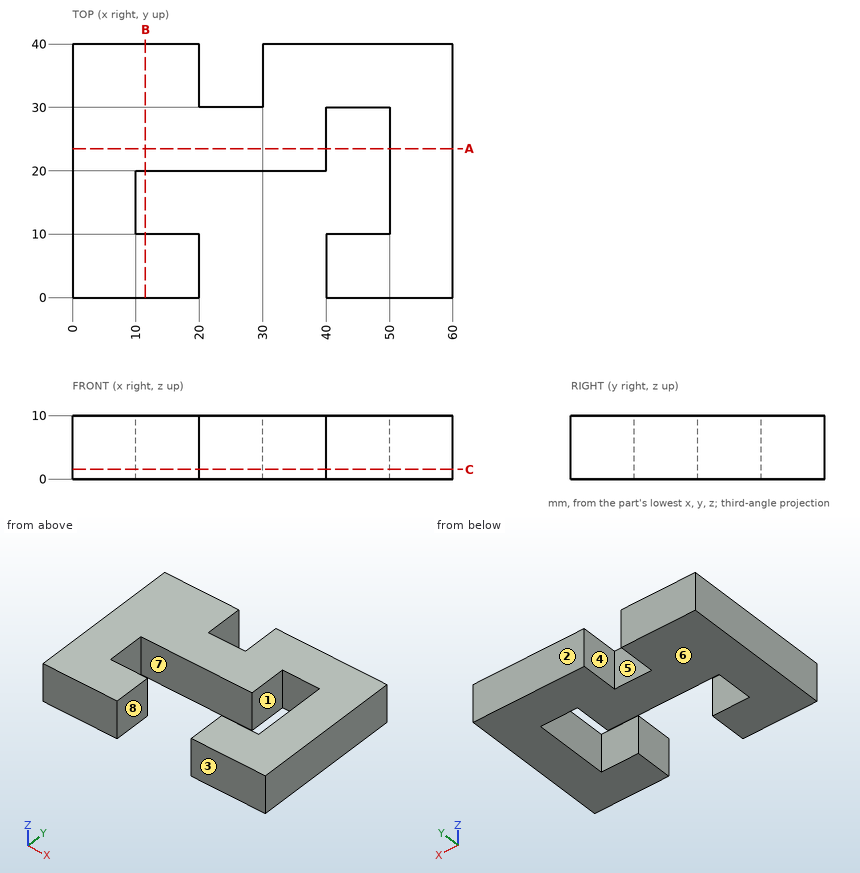
Geometry check sheet. Reference: drawing and pictorial views, mm from the part's lowest x, y, z. A direction names the side the tool comes from. Give positions to 0.01 mm unless a question says otherwise; leave off trailing zeros. Order: outer loops, then holes, each group sorted by start corner. A loop starts at its lowest first (then second) coordinate and runs counter-clockwise, first axis right, second up. Notation, with made-up numbers: M 54.5,-25.75 L 77.5,-25.75 A29 ccw 77.5,1.25 Z; hole C -11,-22.5 d6. An arc over 180 degrees is marked long. Answer as a JSON object with one key per item and string values. Group by question number.
1) Cross-section at C-C (z = 1.5). Enter the section's corners in (x, y), then the cut area to 3 significant figures.
2) Cross-section at A-A (y = 23.5). Enter the section's corners in (x, z), then the cut area to 3 significant figures.
3) Mould release check, pull along Y, two halves, no side actions. Record for the marked faces 1, 2, 3 and 4: released by +Y, released by -Y, zero draft, split by the parting line, or undercut.
4) Cross-section at B-B (x = 11.5). Enter the section's corners in (y, z), then the cut area to 3 significant figures.
5) Depth check by flat-ended pin: pin 1 Ø1 at (x, z) = (22, 8.5) entering from +Y; pin 2 Ø5 at (x, z) = (27.5, 7) entering from -Y. Enter the tip coordinate at first touch or a pass-through.
6) Access from +Z, -Z, +X, -X, +Y, -Y to the whole of each face (thin tool, end or side, straight path). Record for the marked faces 5, 6, 7 and 8.
7) Scan lines: line 1 along Y through (x, z) = (12, 5); line 2 along X through (y, z) = (34, 1.5); line 3 along X through (y, z) = (27.5, 7). Record each from-to range of solid material in increasing order. Write a range as [from, to].
Result sheet:
{
 "1": {"outline": "M 0,0 L 20,0 L 20,10 L 10,10 L 10,20 L 40,20 L 40,30 L 50,30 L 50,10 L 40,10 L 40,0 L 60,0 L 60,40 L 30,40 L 30,30 L 20,30 L 20,40 L 0,40 Z", "area": "1,600 mm2"},
 "2": {"outline": "M 0,0 L 40,0 L 40,10 L 0,10 Z; M 50,0 L 60,0 L 60,10 L 50,10 Z", "area": "500 mm2"},
 "3": {"face 1": "undercut", "face 2": "released by +Y", "face 3": "released by -Y", "face 4": "zero draft"},
 "4": {"outline": "M 0,0 L 10,0 L 10,10 L 0,10 Z; M 20,0 L 40,0 L 40,10 L 20,10 Z", "area": "300 mm2"},
 "5": {"pin 1": "stops at y = 30", "pin 2": "stops at y = 20"},
 "6": {"face 5": "+Z, -Z, +Y", "face 6": "-Z, +X, -X, +Y, -Y", "face 7": "+Z, -Z", "face 8": "+Z, -Z, -Y"},
 "7": {"line 1": "y = [0, 10], [20, 40]", "line 2": "x = [0, 20], [30, 60]", "line 3": "x = [0, 40], [50, 60]"}
}
